Autodesk Inventor part; units mm, degrees
ref_plane "YZ Plane" through (0, 0, 0) normal (1, 0, 0) x (0, 1, 0)
ref_plane "XZ Plane" through (0, 0, 0) normal (0, 1, 0) x (-1, 0, 0)
ref_plane "XY Plane" through (0, 0, 0) normal (0, 0, 1) x (1, 0, 0)
sketch "Sketch1" plane through (0, 0, 0) normal (0, 1, 0) x (-1, 0, 0)
  circle A0 centre (0, 0) radius 85
  line L0 (-55, 64.8074) -> (-55, -64.8074)
  line L1 (23, 75) -> (-35, 75)
  line L2 (-35, 75) -> (-35, 60)
  line L3 (-35, 60) -> (23, 60)
  line L4 (23, 60) -> (23, 75)
  line L5 (-6, 60) -> (-6, 30.4166)
  line L6 (23, -60) -> (-35, -60)
  line L7 (-35, -60) -> (-35, -75)
  line L8 (-35, -75) -> (23, -75)
  line L9 (23, -75) -> (23, -60)
  dimension "d0" = 170
  dimension "d1" = 55
  dimension "d2" = 58
  dimension "d3" = 15
  dimension "d4" = 49
  dimension "d5" = 60
  dimension "d8" = 60
extrude "Extrusion1" add sketch "Sketch1" along normal blind 3 contours A0 L0 picked at (43.6667, 0)
sketch "Sketch2" plane through (0, 0, 0) normal (0, -1, 0) x (1, 0, 0)
  line L0 (-23, 60) -> (-13, 60)
  line L1 (-13, 60) -> (-13, 57)
  line L2 (-13, 57) -> (-23, 57)
  line L3 (-23, 57) -> (-23, 60)
  line L4 (35, 60) -> (25, 60)
  line L5 (25, 60) -> (25, 57)
  line L6 (25, 57) -> (35, 57)
  line L7 (35, 57) -> (35, 60)
  point P0 (0, 0)
  dimension "d9" = 10
  dimension "d10" = 3
  dimension "d11" = 10
  dimension "d12" = 3
extrude "Extrusion2" cut sketch "Sketch2" against normal blind 3
sketch "Sketch3" plane through (0, 0, 0) normal (0, -1, 0) x (1, 0, 0)
  line L0 (18.5, 37) -> (21.5, 37)
  line L1 (21.5, 37) -> (21.5, 27)
  line L2 (21.5, 27) -> (18.5, 27)
  line L3 (18.5, 27) -> (18.5, 37)
  line L4 (35, 57) -> (25, 57)
  line L5 (-13, 60) -> (25, 60) construction
  line L6 (6, 60) -> (6, 41.1412) construction
  point P0 (0, 0)
  dimension "d15" = 3
  dimension "d16" = 10
  dimension "d17" = 20
  dimension "d18" = 12.5
extrude "Extrusion3" cut sketch "Sketch3" against normal blind 3
sketch "Sketch4" plane through (0, 0, 0) normal (0, -1, 0) x (1, 0, 0)
  line L0 (-69.5, 30) -> (-66.5, 30)
  line L1 (-66.5, 30) -> (-66.5, 20)
  line L2 (-66.5, 20) -> (-69.5, 20)
  line L3 (-69.5, 20) -> (-69.5, 30)
  line L4 (55, 64.8074) -> (55, -64.8074)
  line L5 (-69.5, 5) -> (-66.5, 5)
  line L6 (-66.5, 5) -> (-66.5, -5)
  line L7 (-66.5, -5) -> (-69.5, -5)
  line L8 (-69.5, -5) -> (-69.5, 5)
  point P0 (0, 0)
  point P1 (-69.5, 0)
  dimension "d21" = 3
  dimension "d22" = 10
  dimension "d23" = 124.5
  dimension "d24" = 30
  dimension "d25" = 3
  dimension "d26" = 10
extrude "Extrusion4" cut sketch "Sketch4" against normal blind 3
mirror "Mirror1" about plane through (0, 0, 0) normal (0, 0, 1) of "Extrusion3", "Extrusion2", "Extrusion4"
sketch "Sketch5" plane through (0, 0, 0) normal (0, -1, 0) x (1, 0, 0)
  point P0 (0, 0)
properties part number "Mid Plate"
Build history of the part. All positions in model axes, mm. Round coordinates to 2 decimals unless told otherwise and drop trailing zeros. Write each loop counter-clockwise with the first axis right and the second up, starting at its lowest first coordinate (ties: lowest second). Pieces come first, ordered by that corner, then holes. Notation, with made-up numbers: M -10,-26.5 L 45,-26.5 A14 ccw 45,-19.5 Z; hole C 86,-37 d6. An arc over 180 degrees is marked long. Use CSV: the item, a comma, the result in double quotes.
1. Saw through at C-C (y = 2). State how many separate pieces and enclosed holes the cut face has, plus the area to 3 significant figures.
Reply:
separate pieces,"1"
enclosed holes,"7"
area,"18,000 mm²"
2. Saw through at D-D (x = 30). Give the cut face in (y, z), plus the area to 3 significant figures.
Reply:
outline,"M 0,-79.53 L 3,-79.53 L 3,-75 L 0,-75 Z; M 0,-57 L 3,-57 L 3,57 L 0,57 Z; M 0,75 L 3,75 L 3,79.53 L 0,79.53 Z"
area,"369 mm²"
3. Saw through at B-B (x = 0). Give the cut face in (y, z), plus the area to 3 significant figures.
Reply:
outline,"M 0,-85 L 3,-85 L 3,-75 L 0,-75 Z; M 0,-60 L 3,-60 L 3,60 L 0,60 Z; M 0,75 L 3,75 L 3,85 L 0,85 Z"
area,"420 mm²"
4. Wall check: probe 1 along Z at (x, y) = (24, 2.4); probe 2 along Z at (x, y) = (-67.5, 0.7); probe 3 along Z at (x, y) = (-18, 1.1). Give the ranges that are in metal, low to high. Write a range as from..to.
Reply:
probe 1,"z = -81.54..-75, -60..60, 75..81.54"
probe 2,"z = -51.66..-30, -20..-5, 5..20, 30..51.66"
probe 3,"z = -83.07..-75, -57..57, 75..83.07"
5. Saw through at A-A (z = 0). Give the cut face in (x, y).
Reply:
outline,"M -85,0 L -69.5,0 L -69.5,3 L -85,3 Z; M -66.5,0 L 55,0 L 55,3 L -66.5,3 Z"
6. Flat gauge pins, fed straight in: pin 1 (0.9 mm diameter, centred on x = 20, y = 1, fed in from -Z); pin 2 (1.5 mm diameter, centred on x = -67.5, y = 1, fed in from -Z); pin 3 (1 mm diameter, centred on x = -65, y = 2.5, fed in from +Z). Where does each tip first touch, or does it go through?
Reply:
pin 1,"stops at z = -82.72"
pin 2,"stops at z = -52.63"
pin 3,"stops at z = 55.36"
